from build123d import *

# Parameters (mm, degrees)
SKETCH1_W           = 68.7
SKETCH1_H           = 293.84
SKETCH1_R           = 1.7859375
SKETCH1_R_2         = 1.3890625
SKETCH1_R_3         = 11
SKETCH1_W_2         = 26
SKETCH1_H_2         = 72
BOSS_EXTRUDE1_DEPTH = 6.35
SKETCH2_W           = 68.7
SKETCH2_H           = 6.35
BOSS_EXTRUDE2_DEPTH = 6.35


with BuildPart() as part:
    # Sketch1 → Boss-Extrude1 (new body)
    with BuildSketch(Plane.XY):
        with Locations((34.35, -146.92)):
            Rectangle(SKETCH1_W, SKETCH1_H)
        with Locations((50.4128, -189.74)):
            Circle(SKETCH1_R, mode=Mode.SUBTRACT)
        with Locations((50.4128, -245.74)):
            Circle(SKETCH1_R, mode=Mode.SUBTRACT)
        with Locations((34.35, -145.2)):
            Circle(SKETCH1_R_2, mode=Mode.SUBTRACT)
        with Locations((34.35, -103.95)):
            Circle(SKETCH1_R_3, mode=Mode.SUBTRACT)
        with Locations((34.35, -62.7)):
            Circle(SKETCH1_R_2, mode=Mode.SUBTRACT)
        with Locations((31.0878, -210.64)):
            Rectangle(SKETCH1_W_2, SKETCH1_H_2, mode=Mode.SUBTRACT)
    extrude(amount=BOSS_EXTRUDE1_DEPTH)

    # Sketch2 → Boss-Extrude2 (add)
    with BuildSketch(Plane(origin=(0, 0, 0), x_dir=(1, 0, 0), z_dir=(0, 1, 0))):
        with Locations((34.35, -3.175)):
            Rectangle(SKETCH2_W, SKETCH2_H)
    extrude(amount=BOSS_EXTRUDE2_DEPTH)


solid = part.part
The listing builds one solid part. Answer for the finished solid, in the listing's coordinates (mm). A direction names the side the tool comes from. Coordinates: 2 decimals unless noted, no trailing zeros. Loops run counter-clockwise (first coordinate to the right, second up) from the corner with the lowest first, then second, coordinate; pieces in that order, holes last. Notation, with made-up numbers: (-17.75, -33.5) -> (16.25, -33.5) arc R20 cw to (16.25, -11.5) -> close; hole circle Ø6 at (88.5, -22.75). An arc over 180 degrees is marked (long way). Answer in a Markdown table with one row per item. Add a question column.
1. The part is cut by section A-A, the plane z = 4.75. Write down the section's boundary in (x, y), then the cut area to 3 significant figures.
2. The part is cut by section D-D, the plane y = -103.95. Write down the section's boundary in (x, z), then the cut area to 3 significant figures.
3. The part is cut by section B-B, the plane y = -222. Write down the section's boundary in (x, z), then the cut area to 3 significant figures.
4. For faces 1 (the flat face through (31, -174.64, 3)), 2 (the flat face through (68.7, -146, 3)), determine the directions among +Z, -Z, +X, -X, +Y, -Y from which every point of the face is accessible in a straight line to the end or side of a thin tool.
5. Consider line 1 (X direction, y = -189.74, z = 3.75); line 2 (Y direction, x = 34.35, z = 2.25); line 3 (Y direction, x = 19, z = 3). Determine where each line is inside the solid, lowest interval first. Write a range as [from, to].
6. The part is cut by section C-C, the plane x = 40.5. Write down the section's boundary in (y, z), then the cut area to 3 significant figures.
Answer below:
| question | item | result |
|---|---|---|
| 1 | outline | (0, -293.84) -> (68.7, -293.84) -> (68.7, 6.35) -> (0, 6.35) -> close; hole (18.09, -246.64) -> (44.09, -246.64) -> (44.09, -174.64) -> (18.09, -174.64) -> close; hole circle Ø22 at (34.35, -103.95); hole circle Ø2.78 at (34.35, -145.2); hole circle Ø2.78 at (34.35, -62.7); hole circle Ø3.57 at (50.41, -245.74); hole circle Ø3.57 at (50.41, -189.74) |
| 1 | area | 18,300 mm2 |
| 2 | outline | (0, 0) -> (23.35, 0) -> (23.35, 6.35) -> (0, 6.35) -> close; (45.35, 0) -> (68.7, 0) -> (68.7, 6.35) -> (45.35, 6.35) -> close |
| 2 | area | 297 mm2 |
| 3 | outline | (0, 0) -> (18.09, 0) -> (18.09, 6.35) -> (0, 6.35) -> close; (44.09, 0) -> (68.7, 0) -> (68.7, 6.35) -> (44.09, 6.35) -> close |
| 3 | area | 271 mm2 |
| 4 | face 1 | +Z, -Z |
| 4 | face 2 | +Z, -Z, +X, +Y, -Y |
| 5 | line 1 | [0, 18.09], [44.09, 48.63], [52.2, 68.7] |
| 5 | line 2 | [-293.84, -246.64], [-174.64, -146.59], [-143.81, -114.95], [-92.95, -64.09], [-61.31, 6.35] |
| 5 | line 3 | [-293.84, -246.64], [-174.64, 6.35] |
| 6 | outline | (-293.84, 0) -> (-246.64, 0) -> (-246.64, 6.35) -> (-293.84, 6.35) -> close; (-174.64, 0) -> (-113.07, 0) -> (-113.07, 6.35) -> (-174.64, 6.35) -> close; (-94.83, 0) -> (6.35, 0) -> (6.35, 6.35) -> (-94.83, 6.35) -> close |
| 6 | area | 1,330 mm2 |
